Design review of the part built by this model. Coordinates are the model's own, in mm. Coordinates: 2 decimals unless noted, no trailing zeros. Order: outer loops, then holes, each group sorted by start corner. A loop starts at its lowest first (then second) coordinate and runs counter-clockwise, first axis right, second up. Notation, with made-up numbers: (-29.5, 55.25) -> (-23.5, 55.25) arc R30 cw to (-23.5, 77.25) -> close; hole circle Ø8 at (82, 36). An arc over 180 degrees is marked (long way). Write item = value, one per line.
```python
from build123d import *

# Parameters (mm, degrees)
SKETCH_3_W               = 10
SKETCH_3_H               = 4.3
CUT_EXTRUDE_1_DEPTH      = 10
CUT_EXTRUDE_1_DEPTH_BACK = 10
SKETCH_4_R               = 1.6
CUT_EXTRUDE_2_DEPTH      = 23


with BuildPart() as part:
    # Sketch 1 → Revolve 1 (revolve)
    with BuildSketch(Plane.XY):
        Polygon((0, 0), (0, 2), (10, 2), (10, 20), (17, 20), (17, 10), (22, 10), (22, 0), align=None)
    revolve(axis=Axis((0, 0, 0), (1, 0, 0)))

    # Sketch 3 → Cut-Extrude 1 (cut, two sides)
    with BuildSketch(Plane.XY) as cut_extrude_1_sk:
        with Locations((5, 0.15)):
            Rectangle(SKETCH_3_W, SKETCH_3_H)
    extrude(amount=CUT_EXTRUDE_1_DEPTH, mode=Mode.SUBTRACT)
    extrude(cut_extrude_1_sk.sketch, amount=-CUT_EXTRUDE_1_DEPTH_BACK, mode=Mode.SUBTRACT)

    # Sketch 4 → Cut-Extrude 2 (cut)
    with BuildSketch(Plane(origin=(22, 0, 0), x_dir=(0, 0, -1), z_dir=(1, 0, 0))):
        with Locations((0, 8)):
            Circle(SKETCH_4_R)
        with Locations((8, 0)):
            Circle(SKETCH_4_R)
        with Locations((0, -8)):
            Circle(SKETCH_4_R)
        with Locations((-8, 0)):
            Circle(SKETCH_4_R)
    extrude(amount=-CUT_EXTRUDE_2_DEPTH, mode=Mode.SUBTRACT)


solid = part.part
```
(1) We need section C-C (x = 13.25). Write out the cut boundary in (y, z).
Report:
outline = circle Ø40 at (0, 0); hole circle Ø3.2 at (-8, 0); hole circle Ø3.2 at (0, -8); hole circle Ø3.2 at (0, 8); hole circle Ø3.2 at (8, 0)
(2) The part is to be moulded in two halves that separate along Z. For faces 1 (the flat face through (17, -5, 9)), 2 (the cylindrical face through (19.54, -2.17, -9.76)), 3 (the cylindrical face through (16.08, -9.56, 0.35)), say which applies: released by +Z, released by -Z, zero draft, split by the parting line, or undercut.
Report:
face_1 = zero draft
face_2 = split by the parting line
face_3 = undercut
(3) We need section A-A (z = 0). Write out the cut boundary in (x, y).
Report:
outline = (10, -20) -> (17, -20) -> (17, -10) -> (22, -10) -> (22, -9.6) -> (10, -9.6) -> close; (10, -6.4) -> (22, -6.4) -> (22, 6.4) -> (10, 6.4) -> close; (10, 9.6) -> (22, 9.6) -> (22, 10) -> (17, 10) -> (17, 20) -> (10, 20) -> close
(4) For L1, parallel to X at y = -1.5, z = 16; L2, parallel to Y at x = 14.75, z = 8; L3, parallel to Z at x = 13, y = -8.5, list the stretches that pass through material, from the lowest coordinate up.
Report:
L1 = 10 to 17
L2 = -18.33 to -1.6, 1.6 to 18.33
L3 = -18.1 to -1.52, 1.52 to 18.1
(5) Insertion check: pin 1 (8 mm diameter, centred on y = 7, z = 11, fed in from +X); pin 2 (6 mm diameter, centred on y = -14.5, z = -7.5, fed in from +X); pin 3 (2 mm diameter, centred on x = 12.5, y = 3, fed in from -Z); pin 4 (1.9 mm diameter, centred on y = -8, z = 0, fed in from +X). Each pin has a flat end and moves straight along its axis. Give the tip position at first contact, or say it passes through.
Report:
pin_1 = 22
pin_2 = 17
pin_3 = -19.9
pin_4 = through
(6) We need section D-D (y = 8). Write out the cut boundary in (x, z), and give its area (3 significant figures).
Report:
outline = (10, -18.33) -> (17, -18.33) -> (17, -6) -> (22, -6) -> (22, -1.6) -> (10, -1.6) -> close; (10, 1.6) -> (22, 1.6) -> (22, 6) -> (17, 6) -> (17, 18.33) -> (10, 18.33) -> close
area = 278 mm²
